CAD build for the part. Positions are in the model's coordinates, mm. A direction names the side the tool comes from. Give positions to 0.01 mm unless a question says otherwise; leave off trailing zeros. Loops run counter-clockwise (first coordinate to the right, second up) from the corner with the lowest first, then second, coordinate; pieces in that order, holes last. Notation, with made-up numbers: (20, 3) - (46, 3) arc R22 ccw to (46, 12) - close; hole circle Ø1 at (44.5, 12.5). An arc over 180 degrees is marked (long way). Return JSON: item names as keys, results as strings.
Autodesk Inventor part; units mm, degrees
ref_plane "YZ Plane" through (0, 0, 0) normal (1, 0, 0) x (0, 1, 0)
ref_plane "XZ Plane" through (0, 0, 0) normal (0, 1, 0) x (-1, 0, 0)
ref_plane "XY Plane" through (0, 0, 0) normal (0, 0, 1) x (1, 0, 0)
sketch "Skizze1" plane through (0, 0, 0) normal (0, 0, 1) x (1, 0, 0)
  line L0 (-36.1506, 26.4082) -> (43.8494, 26.4082)
  line L1 (43.8494, 26.4082) -> (43.8494, -13.5918)
  line L2 (43.8494, -13.5918) -> (-36.1506, -13.5918)
  line L3 (-36.1506, -13.5918) -> (-36.1506, 26.4082)
  line L4 (-34.9406, 25.1642) -> (-33.7406, 25.1642)
  line L5 (-33.7406, 25.1642) -> (-33.7406, -12.3818)
  line L6 (-33.7406, -12.3818) -> (-34.9406, -12.3818)
  line L7 (-34.9406, -12.3818) -> (-34.9406, 25.1642)
  line L8 (41.4394, 23.5568) -> (42.6394, 23.5568)
  line L9 (42.6394, 23.5568) -> (42.6394, -12.3818)
  line L10 (42.6394, -12.3818) -> (41.4394, -12.3818)
  line L11 (41.4394, -12.3818) -> (41.4394, 23.5568)
  line L12 (-32.9506, 26.4082) -> (40.6494, 26.4082)
  line L13 (40.6494, 26.4082) -> (40.6494, 4.4082)
  line L14 (40.6494, 4.4082) -> (-32.9506, 4.4082)
  line L15 (-32.9506, 4.4082) -> (-32.9506, 26.4082)
  line L16 (-26.1506, -11.1818) -> (33.8494, -11.1818)
  line L17 (33.8494, -11.1818) -> (33.8494, -12.3818)
  line L18 (33.8494, -12.3818) -> (-26.1506, -12.3818)
  line L19 (-26.1506, -12.3818) -> (-26.1506, -11.1818)
  line L20 (42.6394, 0.4082) -> (41.4394, 0.4082)
  line L21 (41.4394, 0.4082) -> (41.4394, 6.4082)
  line L22 (41.4394, 6.4082) -> (42.6394, 6.4082)
  line L23 (42.6394, 6.4082) -> (42.6394, 0.4082)
  line L24 (-33.7406, 0.4082) -> (-34.9406, 0.4082)
  line L25 (-34.9406, 0.4082) -> (-34.9406, 6.4082)
  line L26 (-34.9406, 6.4082) -> (-33.7406, 6.4082)
  line L27 (-33.7406, 6.4082) -> (-33.7406, 0.4082)
  point P0 (0, 0)
  point P1 (-32.9506, 15.4082)
  point P2 (42.0394, -12.3818)
  point P3 (33.8494, -11.7818)
  point P4 (-26.1506, -11.7818)
  point P5 (42.0394, 0.4082)
  point P6 (42.0394, 6.4082)
  point P7 (-34.3406, 0.4082)
  point P8 (-34.3406, 6.4082)
  dimension "d0" = 80
  dimension "d1" = 40
  dimension "d2" = 1.21
  dimension "d3" = 1.21
  dimension "d4" = 35.9386
  dimension "d5" = 1.2
  dimension "d6" = 1.2
  dimension "d7" = 18
  dimension "d8" = 3.2
  dimension "d9" = 3.2
  dimension "d10" = 1.21
  dimension "d11" = 1.21
  dimension "d12" = 1.2
  dimension "d13" = 10
  dimension "d14" = 10
  dimension "d15" = 14
  dimension "d16" = 6
  dimension "d17" = 14
  dimension "d18" = 6
extrude "Extrusion1" add sketch "Skizze1" along normal blind 1.5 contours L0 L15 L14 L13 L1 L2 L3
extrude "Extrusion2" add sketch "Skizze1" along normal blind 3 contours L4 L5 L26 L7 | L24 L5 L6 L7 | L8 L9 L22 L11 | L20 L9 L10 L11 | L16 L17 L18 L19
extrude "Extrusion3" add sketch "Skizze1" along normal blind 7 contours L26 L5 L24 L7 | L22 L9 L20 L11
sketch "Skizze2" plane through (42.6394, -12.3818, 1.5) normal (1, 0, 0) x (0, 0, -1)
  circle A0 centre (-3, 15.79) radius 1
  line L0 (0, -1.21) -> (0, 38.79)
  line L1 (1.5, -1.21) -> (0, -1.21)
  point P0 (1.5, 12.3818)
  point P1 (0.75, -1.21)
  dimension "d25" = 2
  dimension "d26" = 3
  dimension "d27" = 17
extrude "Extrusion4" cut sketch "Skizze2" against normal through all
properties part number "Konsole_Deckel"
1. Drill centre lines: probe 1 along Y at (x, z) = (41.7, 4.5); probe 2 along X at (y, z) = (12, 0.5); probe 3 along X at (y, z) = (5.5, 6). Where is each one in solid material? Low to high.
Values follow:
{"probe 1": "y = 0.41 to 2.41, 4.41 to 6.41", "probe 2": "x = -36.15 to -32.95, 40.65 to 43.85", "probe 3": "x = -34.94 to -33.74, 41.44 to 42.64"}
2. Cut at C-C, the plane x = 31. Write the cut outline in (y, z), plus the area to 3 significant figures.
Values follow:
{"outline": "(-13.59, 0) - (4.41, 0) - (4.41, 1.5) - (-11.18, 1.5) - (-11.18, 3) - (-12.38, 3) - (-12.38, 1.5) - (-13.59, 1.5) - close", "area": "28.8 mm²"}
3. Cut at B-B, the plane y = 9.5. Write the cut outline in (x, z), plus the area to 3 significant figures.
Values follow:
{"outline": "(-36.15, 0) - (-32.95, 0) - (-32.95, 1.5) - (-33.74, 1.5) - (-33.74, 3) - (-34.94, 3) - (-34.94, 1.5) - (-36.15, 1.5) - close; (40.65, 0) - (43.85, 0) - (43.85, 1.5) - (42.64, 1.5) - (42.64, 3) - (41.44, 3) - (41.44, 1.5) - (40.65, 1.5) - close", "area": "13.2 mm²"}
4. Drop flat-ended pins along their axis: P1, Ø1, axis at x = 42, z = 2.5, coming from the +Y side; P2, Ø0.8, axis at x = -4, z = 2.5, coming from the -Y side; P3, Ø0.6, axis at x = -34.5, y = 17.5, coming from the +Z side. Give the stop position or say it passes through.
Values follow:
{"P1": "stops at y = 23.56", "P2": "stops at y = -12.38", "P3": "stops at z = 3"}
5. Which spindle directions (+Z, -Z, +X, -X, +Y, -Y) get a long thin tool onto all of the face, cutting with end or side? Do faces 1 (the face through (42.639, 6, 3)), 2 (the face through (41.439, 5, 3)), 3 (the face through (-32.951, 15, 1)). Say none if no direction does.
Values follow:
{"face 1": "+Z, +X, +Y, -Y", "face 2": "+Z, +Y, -Y", "face 3": "+Z, -Z, +Y"}
6. Pull direction X, two halves, no side cores. Call faces 4 (the face through (-35, 26.408, 1)), 5 (the face through (3, -2, 1.5)), 6 (the face through (40.649, 16, 1)), 7 (the face through (43.849, 7, 1)): +X half, -X half, draft (parallel to the pull), parting line (faces both ways), or undercut.
Values follow:
{"face 4": "draft", "face 5": "undercut", "face 6": "undercut", "face 7": "+X half"}
7. Cut at A-A, the plane z = 4.5. Write the cut outline in (x, y), plus the area to 3 significant figures.
Values follow:
{"outline": "(-34.94, 0.41) - (-33.74, 0.41) - (-33.74, 2.41) - (-34.94, 2.41) - close; (-34.94, 4.41) - (-33.74, 4.41) - (-33.74, 6.41) - (-34.94, 6.41) - close; (41.44, 0.41) - (42.64, 0.41) - (42.64, 2.41) - (41.44, 2.41) - close; (41.44, 4.41) - (42.64, 4.41) - (42.64, 6.41) - (41.44, 6.41) - close", "area": "9.60 mm²"}
8. Cut at D-D, the plane y = -7.5. Write the cut outline in (x, z), plus the area to 3 significant figures.
Values follow:
{"outline": "(-36.15, 0) - (43.85, 0) - (43.85, 1.5) - (42.64, 1.5) - (42.64, 3) - (41.44, 3) - (41.44, 1.5) - (-33.74, 1.5) - (-33.74, 3) - (-34.94, 3) - (-34.94, 1.5) - (-36.15, 1.5) - close", "area": "124 mm²"}
